```python
from build123d import *

# Parameters (mm, degrees)
BOSS_EXTRUDE1_DEPTH         = 609.6
FILLET1_R                   = 2.54
F_1_4_CLEARANCE_HOLE1_D     = 6.5278
F_1_4_CLEARANCE_HOLE1_DEPTH = 22.352
F_1_4_CLEARANCE_HOLE1_TIP   = 1.961148974


with BuildPart() as part:
    # Sketch1 → Boss-Extrude1 (new body)
    with BuildSketch(Plane(origin=(0, 0, 0), x_dir=(0, 0, -1), z_dir=(1, 0, 0))):
        Polygon((0, 0), (-12.7, 0), (-12.7, 12.7), (-6.35, 12.7), (-6.35, 9.525), (-9.525, 9.525), (-9.525, 3.175), (0, 3.175), align=None)
    boss_extrude1 = extrude(amount=BOSS_EXTRUDE1_DEPTH)

    # Mirror1: Boss-Extrude1 across plane
    add(boss_extrude1.mirror(Plane(origin=(609.6, 3.175, 0), x_dir=(1, 0, 0), z_dir=(0, 0, 1))))

    # Fillet1
    fillet1_edges = [part.edges().sort_by_distance(p)[0] for p in [
        (304.8, 0, 12.7),
        (304.8, 12.7, 12.7),
        (304.8, 0, -12.7),
        (304.8, 12.7, -12.7),
    ]]
    fillet(fillet1_edges, radius=FILLET1_R)

    # 1/4 Clearance Hole1
    with Locations(Plane(origin=(0, 3.175, 0), x_dir=(1, 0, 0), z_dir=(0, 1, 0))):
        with Locations((25.4, 0), (533.4, 0)):
            Hole(F_1_4_CLEARANCE_HOLE1_D / 2, depth=F_1_4_CLEARANCE_HOLE1_DEPTH)
            with Locations((0, 0, -(F_1_4_CLEARANCE_HOLE1_DEPTH + F_1_4_CLEARANCE_HOLE1_TIP / 2))):  # 118° drill point
                Cone(0, F_1_4_CLEARANCE_HOLE1_D / 2, F_1_4_CLEARANCE_HOLE1_TIP, mode=Mode.SUBTRACT)


solid = part.part
```
Can you work these out from the model? Positions are in its coordinate system, mm. Give positions to 0.01 mm unless a question says otherwise; leave off trailing zeros. Order: outer loops, then holes, each group sorted by start corner. A loop starts at its lowest first (then second) coordinate and runs counter-clockwise, first axis right, second up. Notation, with made-up numbers: M -18,-13.5 L 8,-13.5 A33 ccw 8,23.5 Z; hole C 2.5,67 d11. An arc over 180 degrees is marked long. Write item = value, one per line. Start each with the question number.
Q1. Suppose I cut it at A-A (y = 5.5). Write out the boundary of the cut face in (x, z) (3 decimals).
Q2. Suppose I cut it at B-B (x = 77). Write out the boundary of the cut face in (y, z) (3 decimals), plus the area to 3 significant figures.
Q3. Will these pins go through, and if not, where does the flat tip stop? pin 1 Ø4 at (x, z) = (97, 3.5) entering from +Y (3 decimals); pin 2 Ø1 at (x, y) = (389, 11.5) entering from +Z.
Q4. We'd pull the mould along Y, two halves only. Please class faces 1 (the flat face through (301, 3.175, 0)), 2 (the flat face through (0, 2, 0)), 3 (the flat face through (301, 0, 0)): pulls with the +Y half, pulls with the -Y half, needs draft (parallel to the pull), parting line crosses it, or undercut.
Q5. I need wall thicknesses on probe 1 along Z at (x, y) = (533.4, 1.9); probe 2 along Y at (x, z) = (317.5, 6.5) (3 decimals); probe 3 along Z at (x, y) = (98, 10.25). Which ranges of each line are inside material? Lowest first, please. Write a range as [from, to].
Check result:
q1.outline = M 0,-12.7 L 609.6,-12.7 L 609.6,-9.525 L 0,-9.525 Z; M 0,9.525 L 609.6,9.525 L 609.6,12.7 L 0,12.7 Z
q2.outline = M 0,-10.16 A2.54 ccw 2.54,-12.7 L 10.16,-12.7 A2.54 ccw 12.7,-10.16 L 12.7,-6.35 L 9.525,-6.35 L 9.525,-9.525 L 3.175,-9.525 L 3.175,9.525 L 9.525,9.525 L 9.525,6.35 L 12.7,6.35 L 12.7,10.16 A2.54 ccw 10.16,12.7 L 2.54,12.7 A2.54 ccw 0,10.16 Z
q2.area = 156 mm2
q3.pin_1 = 3.175
q3.pin_2 = 12.56
q4.face_1 = undercut
q4.face_2 = needs draft
q4.face_3 = pulls with the -Y half
q5.probe_1 = [-12.62, -3.26], [3.26, 12.62]
q5.probe_2 = [0, 3.175], [9.525, 12.7]
q5.probe_3 = [-12.7, -6.35], [6.35, 12.7]
